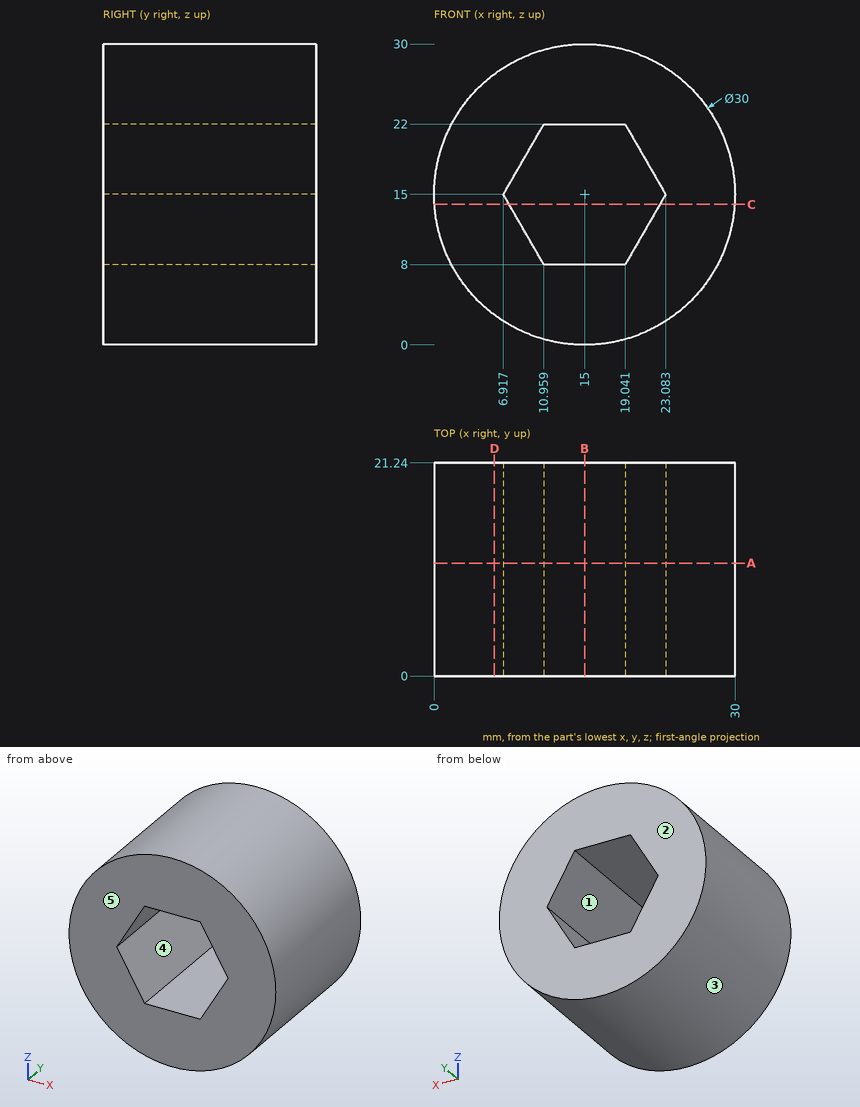
The figure shows three views and two pictorial views of one solid part (mm, origin at its lowest corner). Answer the questions. A direction names the side the tool comes from. Round coordinates to 2 decimals unless told otherwise and drop trailing zeros. Order: outer loops, then holes, each group sorted by start corner. A loop starts at its lowest first (then second) coordinate and runs counter-clockwise, first axis right, second up. Notation, with made-up numbers: (80.25, 78.5) -> (110.25, 78.5) arc R27 ccw to (110.25, 110.5) -> close; hole circle Ø4 at (3, 43.5). An arc over 180 degrees is marked (long way). Put each result on its own line as item: value.
Q1. Which of the six approach directions +Z, -Z, +X, -X, +Y, -Y give full straight-line access (tool end or side, diameter ignored) to the marked faces 1 and 2?
Results list:
face 1: +Y, -Y
face 2: +Z, -Z, +X, -X, +Y
Q2. Each of these flat-tipped pins is pushed along its axis until it touches: P1, Ø10, axis at y = 18.5, z = 7.5, coming from the -X side; P2, Ø10, axis at y = 18, z = 5, coming from the -X side; P3, Ø12, axis at x = 7.5, y = 17.5, coming from the -Z side (1 decimal). Where does it stop, or does it pass through?
Results list:
P1: x = 0.21
P2: x = 0.86
P3: z = 0.1
Q3. Section D-D, the plane x = 6 is taken. Write down the section's boundary in (y, z), and give its area (3 significant figures).
Results list:
outline: (0, 3) -> (21.24, 3) -> (21.24, 27) -> (0, 27) -> close
area: 510 mm^2
Q4. Determine the mould class of the marked faces 3, 4 and 5 for opening direction Z: pulls with the +Z half, pulls with the -Z half, needs draft (parallel to the pull), parting line crosses it, or undercut.
Results list:
face 3: parting line crosses it
face 4: undercut
face 5: needs draft
Q5. Section C-C, the plane z = 14 is taken. Write down the section's boundary in (x, y) (1 decimal).
Results list:
outline: (0, 0) -> (7.5, 0) -> (7.5, 21.2) -> (0, 21.2) -> close; (22.5, 0) -> (30, 0) -> (30, 21.2) -> (22.5, 21.2) -> close
Q6. Section A-A, the plane y = 11.25 is taken. Write down the section's boundary in (x, z), and give its area (3 significant figures).
Results list:
outline: circle Ø30 at (15, 15); hole (6.92, 15) -> (10.96, 8) -> (19.04, 8) -> (23.08, 15) -> (19.04, 22) -> (10.96, 22) -> close
area: 537 mm^2
Q7. Consider line 1 along Z through (x, y) = (15.25, 17); line 2 along X through (y, z) = (11.25, 9.75); line 3 along X through (y, z) = (6, 19.5) (1 decimal). Determine where each line is inside the solid, lowest interval first.
Results list:
line 1: 0 to 8, 22 to 30
line 2: 0.95 to 9.95, 20.05 to 29.05
line 3: 0.7 to 9.5, 20.5 to 29.3
Q8. Section B-B, the plane x = 15 is taken. Write down the section's boundary in (y, z), and give its area (3 significant figures).
Results list:
outline: (0, 0) -> (21.24, 0) -> (21.24, 8) -> (0, 8) -> close; (0, 22) -> (21.24, 22) -> (21.24, 30) -> (0, 30) -> close
area: 340 mm^2
